Build history of the part. All positions in model axes, mm. Coordinates: 2 decimals unless noted, no trailing zeros. Write each loop counter-clockwise with the first axis right and the second up, starting at its lowest first coordinate (ties: lowest second). Pieces come first, ordered by that corner, then holes. Notation, with made-up numbers: (9.25, -1.75) -> (36.25, -1.75) arc R33 cw to (36.25, 33.25) -> close; hole circle Ø7 at (81.5, 45). An arc over 180 degrees is marked (long way). Write each question's results on one line, items separated by ' | '. Start each with the question number.
Q1. Drill centre lines: line 1 (X direction, y = 344, z = 2.55); line 2 (Y direction, x = 388, z = 4.85); line 3 (X direction, y = -348.5, z = 5). Where is each one in solid material? Low to high.
Q2. Drop flat-ended pins along their axis: pin 1 Ø2 at (x, y) = (-103.5, 301) entering from -Z; pin 2 Ø3 at (y, z) = (380, 1.5) entering from -X. Give the stop position or say it passes through.
Q3. Saw through at A-A on z = 3.3. Give the cut face in (x, y).
from build123d import *

# Parameters (mm, degrees)
SKETCH1_W           = 860
SKETCH1_H           = 780
BOSS_EXTRUDE1_DEPTH = 6
SKETCH2_W           = 60
SKETCH2_H           = 60
CUT_EXTRUDE1_DEPTH  = 6
CHAMFER1_SIZE       = 40


with BuildPart() as part:
    # Sketch1 → Boss-Extrude1 (new body)
    with BuildSketch(Plane.XY):
        Rectangle(SKETCH1_W, SKETCH1_H)
    extrude(amount=BOSS_EXTRUDE1_DEPTH)

    # Sketch2 → Cut-Extrude1 (cut)
    with BuildSketch(Plane.XY.offset(6)):
        with Locations((-400, 360)):
            Rectangle(SKETCH2_W, SKETCH2_H)
        with Locations((400, 360)):
            Rectangle(SKETCH2_W, SKETCH2_H)
        with Locations((400, -360)):
            Rectangle(SKETCH2_W, SKETCH2_H)
        with Locations((-400, -360)):
            Rectangle(SKETCH2_W, SKETCH2_H)
    extrude(amount=-CUT_EXTRUDE1_DEPTH, mode=Mode.SUBTRACT)

    # Chamfer1
    chamfer1_edges = [part.edges().sort_by_distance(p)[0] for p in [
        (-370, -330, 3),
        (370, -330, 3),
        (370, 330, 3),
        (-370, 330, 3),
    ]]
    chamfer(chamfer1_edges, length=CHAMFER1_SIZE)


solid = part.part
Returned:
1) line 1: x = -396 to 396 | line 2: y = -352 to 352 | line 3: x = -391.5 to 391.5
2) pin 1: stops at z = 0 | pin 2: stops at x = -370
3) outline: (-430, -330) -> (-410, -330) -> (-370, -370) -> (-370, -390) -> (370, -390) -> (370, -370) -> (410, -330) -> (430, -330) -> (430, 330) -> (410, 330) -> (370, 370) -> (370, 390) -> (-370, 390) -> (-370, 370) -> (-410, 330) -> (-430, 330) -> close
